from build123d import *

# Parameters (mm, degrees)
F1_DEPTH = 1.27
F3_DEPTH = 12.7
F6_DEPTH = 1.778


with BuildPart() as f1:
    # F0 (on Top) → F1 (new body, symmetric)
    with BuildSketch(Plane.XY):
        with BuildLine():
            Line((0, 1.524), (0, 0))
            Line((0, 0), (12.7, 0))
            Line((12.7, 0), (12.7, -2.54))
            Line((12.7, -2.54), (4.572, -2.54))
            Line((4.572, -2.54), (4.572, -4.572))
            Line((4.572, -4.572), (12.5717104354, -4.572))
            ThreePointArc((12.5717104354, -4.572), (15.7940682602, -1.0438103752), (11.7644204026, 1.524))
            Line((11.7644204026, 1.524), (0, 1.524))
        make_face()
    extrude(amount=F1_DEPTH, both=True)

    # F2 (on face) → F3 (join, through all)
    with BuildSketch(Plane(origin=(0, 0, 0), x_dir=(0, -1, 0), z_dir=(-1, 0, 0))):
        Polygon((0.762, 0), (0, 0.508), (0, -0.508), align=None)
    extrude(amount=-F3_DEPTH)

    # F5 (on face) → F6 (join)
    with BuildSketch(Plane(origin=(3.81, 0, 0), x_dir=(0, -1, 0), z_dir=(-1, 0, 0))):
        Polygon((-4.064, -1.27), (-1.524, -1.27), (-1.524, 1.27), align=None)
    extrude(amount=-F6_DEPTH)


solid = f1.part
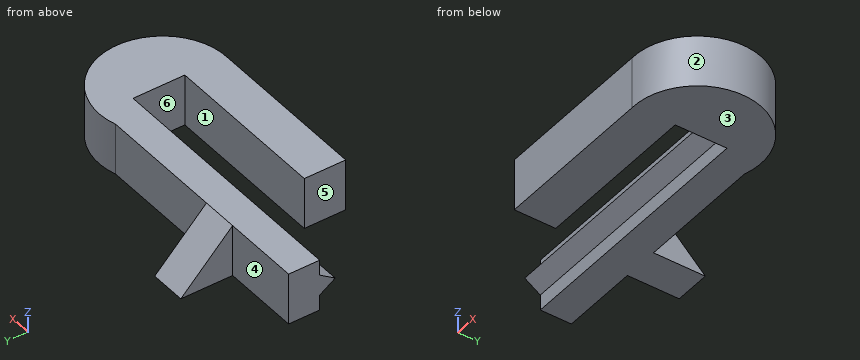
CAD build for the part. Positions are in the model's coordinates, mm. Face numbers are marked on the shaded views. A direction names the side the tool comes from. Round coordinates to 2 decimals unless told otherwise and drop trailing zeros. Write each loop counter-clockwise with the first axis right and the second up, starting at its lowest first coordinate (ties: lowest second). Pieces come first, ordered by that corner, then holes.
(1) Probe line 1 along Y through (x, z) = (6, 1.1); line 2 along Y through (x, z) = (2.75, 0.9); line 3 along Y through (x, z) = (12.25, -0.55). List the from-to ranges inside material, lowest first.
(2) Drop flat-ended pins along their axis: P1, Ø1.3, axis at x = 10, z = 0, coming from the +Y side; P2, Ø0.8, axis at y = -1.5, z = 0, coming from the -X side; P3, Ø1.5, axis at x = 4.5, z = 0, coming from the +Y side. Give the stop position or say it passes through.
(3) Slice it at D-D, the plane z = -0.9. Write the cut outline in (x, y), and give its area (3 significant figures).
(4) Slice it at A-A, the plane x = 2.25. Write the cut outline in (y, z), and give its area (3 significant figures).
(5) Slice it at B-B, the plane z = 1.1. Write the cut outline in (x, y), and give its area (3 significant figures).
(6) 3-axis set-ups, long thin cutter, end or side, ignore diameter. For the marked faces 4, 5 and 6: which of +Z, -Z, +X, -X, +Y, -Y reach the whole face in a straight line?
(7) Mould opens along Y. For the marked faces 1, 2 and 3 say: pulls with the +Y half, pulls with the -Y half, needs draft (parallel to the pull), parting line crosses it, or undercut.
(8) Slice it at C-C, the plane y = -3.5. Write the cut outline in (x, z).
From the geometry:
1. line 1: y = -4.57 to -2.54, 0 to 1.52
1. line 2: y = 0 to 1.52
1. line 3: y = -4.57 to -2.54, 0 to 1.63
2. P1: stops at y = 1.52
2. P2: stops at x = 12.7
2. P3: stops at y = 3.54
3. outline: (0, 0) - (12.7, 0) - (12.7, -2.54) - (4.57, -2.54) - (4.57, -4.57) - (12.57, -4.57) arc R3.12 ccw (long way) to (11.76, 1.52) - (5.59, 1.52) - (5.59, 3.69) - (3.81, 3.69) - (3.81, 1.52) - (0, 1.52) - close
3. area: 55.1 mm2
4. outline: (-0.76, 0) - (0, -0.51) - (0, -1.27) - (1.52, -1.27) - (1.52, 1.27) - (0, 1.27) - (0, 0.51) - close
4. area: 4.26 mm2
5. outline: (0, 0) - (12.7, 0) - (12.7, -2.54) - (4.57, -2.54) - (4.57, -4.57) - (12.57, -4.57) arc R3.12 ccw (long way) to (11.76, 1.52) - (5.59, 1.52) - (5.59, 1.69) - (3.81, 1.69) - (3.81, 1.52) - (0, 1.52) - close
5. area: 51.6 mm2
6. face 4: +Z, -Z, -X, +Y
6. face 5: +Z, -Z, -X, -Y
6. face 6: -X
7. face 1: undercut
7. face 2: parting line crosses it
7. face 3: needs draft
8. outline: (4.57, -1.27) - (15.06, -1.27) - (15.06, 1.27) - (4.57, 1.27) - close
